from build123d import *

# Parameters (mm, degrees)
SKETCH1_R         = 4.0005
EXTRUDE1_DEPTH    = 2.159
SKETCH2_R         = 2.032
EXTRUDE2_DEPTH    = 8.89
SKETCH3_W         = 5.08
SKETCH3_H         = 0.508
EXTRUDE3_DEPTH    = 1.016
CIRPATTERN1_COUNT = 2
CIRPATTERN1_ANGLE = 90
CHAMFER1_SIZE     = 1.9558


with BuildPart() as part:
    # Sketch1 → Extrude1 (new body)
    with BuildSketch(Plane.XY):
        Circle(SKETCH1_R)
    extrude(amount=EXTRUDE1_DEPTH)

    # Sketch2 → Extrude2 (add)
    with BuildSketch(Plane.XY.offset(2.159)):
        Circle(SKETCH2_R)
    extrude(amount=EXTRUDE2_DEPTH)

    # Sketch3 → Extrude3 (cut)
    with BuildSketch(Plane(origin=(0, 0, 0), x_dir=(-1, 0, 0), z_dir=(0, 0, -1))):
        Rectangle(SKETCH3_W, SKETCH3_H)
    extrude3 = extrude(amount=-EXTRUDE3_DEPTH, mode=Mode.SUBTRACT)

    # CirPattern1: Extrude3 ×2 about axis
    cirpattern1_axis = Axis((0, 0, 0), (0, 0, -1))
    for i in range(1, CIRPATTERN1_COUNT):
        add(extrude3.rotate(cirpattern1_axis, i * CIRPATTERN1_ANGLE / (CIRPATTERN1_COUNT - 1)), mode=Mode.SUBTRACT)

    # Chamfer1
    chamfer1_edges = [part.edges().sort_by_distance(p)[0] for p in [
        (-4.0005, 0, 2.159),
    ]]
    chamfer(chamfer1_edges, length=CHAMFER1_SIZE)


solid = part.part
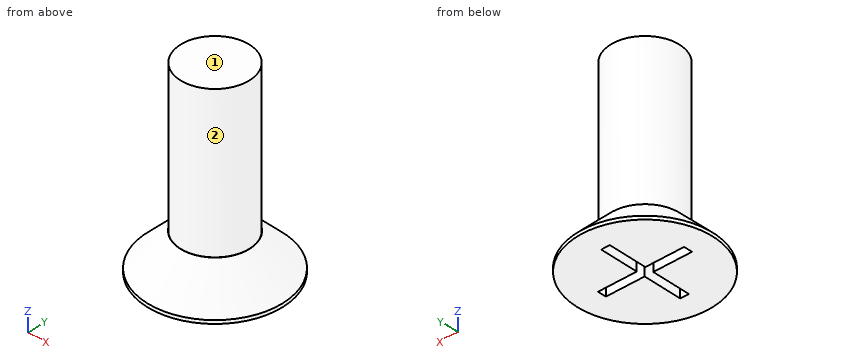
Build history of the part. All positions in model axes, mm. Face numbers are marked on the shaded views. A direction names the side the tool comes from. Coordinates: 2 decimals unless noted, no trailing zeros. Write each loop counter-clockwise with the first axis right and the second up, starting at its lowest first coordinate (ties: lowest second). Pieces come first, ordered by that corner, then holes.
(1) Cut at C-C on z = 3.75. List the corners of the cut face in (x, y).
(2) 3-axis set-ups, long thin cutter, end or side, ignore diameter. For the marked faces 1 and 2: which of +Z, -Z, +X, -X, +Y, -Y reach the whole face in a straight line?
(3) Pin check, flat tips, straight feed: pin 1 Ø3 at (x, z) = (1.5, 9.5) entering from -Y; pin 2 Ø0.8 at (y, z) = (-2, 0.5) entering from -X; pin 3 Ø0.8 at (x, z) = (2, 0.5) entering from +Y. Stop position of each tip, or through.
(4) Cut at D-D on z = 2. List the corners of the cut face in (x, y), and give its area (3 significant figures).
(5) Drill centre lines: line 1 (X direction, y = 2, z = 0.5); line 2 (Y direction, x = -0.75, z = 9); line 3 (Y direction, x = -1.5, z = 3.5). Where is each one in solid material? Low to high.
Working result:
1. outline: circle Ø4.06 at (0, 0)
2. face 1: +Z, +X, -X, +Y, -Y
2. face 2: +Z
3. pin 1: stops at y = -2.03
3. pin 2: stops at x = -3.61
3. pin 3: stops at y = 3.61
4. outline: circle Ø4.41 at (0, 0)
4. area: 15.3 mm2
5. line 1: x = -3.12 to -0.25, 0.25 to 3.12
5. line 2: y = -1.89 to 1.89
5. line 3: y = -1.37 to 1.37
